```python
from build123d import *
from build123d.topology import SkipClean

# Parameters (mm, degrees)
BOSS_EXTRUDE1_DEPTH      = 1.3
BOSS_EXTRUDE2_DEPTH      = 10
BOSS_EXTRUDE2_DEPTH_BACK = 2.3
SKETCH2_R                = 1.79
SKETCH4_W                = 8.8
SKETCH4_H                = 1.3
BOSS_EXTRUDE4_DEPTH      = 2.4
SKETCH3_W                = 8.8
SKETCH3_H                = 10
BOSS_EXTRUDE3_DEPTH      = 1.3
FILLET4_R                = 1.3
FILLET6_R                = 1
SKETCH5_R                = 1.5
CUT_EXTRUDE1_DEPTH       = 2.4
FILLET7_R                = 1
FILLET4_OF_MIRROR1_R     = 1.3
FILLET6_OF_MIRROR1_R     = 1
FILLET7_OF_MIRROR1_R     = 1
BOSS_EXTRUDE5_START      = 7
SKETCH6_W                = 18
SKETCH6_H                = 70
SKETCH6_R                = 1.5
BOSS_EXTRUDE5_DEPTH      = 7
SKETCH9_R                = 4
CUT_EXTRUDE3_DEPTH       = 3
CUT_EXTRUDE4_DEPTH       = 72.965296541


with BuildPart() as part:
    # Sketch1 → Boss-Extrude1 (new body)
    with BuildSketch(Plane.XY):
        with BuildLine():
            Line((-4.7625, -4.5), (4.7625, -4.5))
            ThreePointArc((4.7625, -4.5), (8.887505516, 1.798424168), (1.465384615, 3.062520227))
            ThreePointArc((1.465384615, 3.062520227), (0, 2.423640328), (-1.465384615, 3.062520227))
            ThreePointArc((-1.465384615, 3.062520227), (-8.887505516, 1.798424168), (-4.7625, -4.5))
        make_face()
    boss_extrude1 = extrude(amount=BOSS_EXTRUDE1_DEPTH)

    # Sketch2 → Boss-Extrude2 (add, two sides: drawn at the far end of the back side and taken through both)
    with BuildSketch(Plane.XY.offset(1.3).offset(-BOSS_EXTRUDE2_DEPTH_BACK)):
        with Locations((-4.7625, 0)):
            Circle(SKETCH2_R)
        with Locations((4.7625, 0)):
            Circle(SKETCH2_R)
    extrude(amount=BOSS_EXTRUDE2_DEPTH + BOSS_EXTRUDE2_DEPTH_BACK)

    # Sketch4 → Boss-Extrude4 (add)
    with BuildSketch(Plane.XZ.offset(4.5)):
        with Locations((0, 0.65)):
            Rectangle(SKETCH4_W, SKETCH4_H)
    boss_extrude4 = extrude(amount=BOSS_EXTRUDE4_DEPTH)

    # Sketch3 → Boss-Extrude3 (add)
    with BuildSketch(Plane.XZ.offset(6.9)):
        with Locations((0, -3.7)):
            Rectangle(SKETCH3_W, SKETCH3_H)
    boss_extrude3 = extrude(amount=-BOSS_EXTRUDE3_DEPTH)

    # Fillet4
    fillet4_edges = [part.edges().sort_by_distance(p)[0] for p in [
        (0, -6.9, 1.3),
    ]]
    fillet(fillet4_edges, radius=FILLET4_R)

    # Fillet6
    fillet6_edges = [part.edges().sort_by_distance(p)[0] for p in [
        (0, -5.6, 0),
    ]]
    fillet(fillet6_edges, radius=FILLET6_R)

    # Sketch5 → Cut-Extrude1 (cut)
    with BuildSketch(Plane.XZ.offset(6.9)):
        with Locations(Location((0, -4.35, 0), (0, 0, 270))):
            Circle(SKETCH5_R)
    cut_extrude1 = extrude(amount=-CUT_EXTRUDE1_DEPTH, mode=Mode.SUBTRACT)

    # Fillet7
    fillet7_edges = [part.edges().sort_by_distance(p)[0] for p in [
        (-4.4, -6.25, -8.7),
        (4.4, -6.25, -8.7),
    ]]
    fillet(fillet7_edges, radius=FILLET7_R)

    # Mirror1: Boss-Extrude1, Boss-Extrude4, Boss-Extrude3, Cut-Extrude1 across plane
    add(boss_extrude1.mirror(Plane(origin=(0, 0, 5.15), x_dir=(1, 0, 0), z_dir=(0, 0, -1))))
    add(boss_extrude4.mirror(Plane(origin=(0, 0, 5.15), x_dir=(1, 0, 0), z_dir=(0, 0, -1))))
    add(boss_extrude3.mirror(Plane(origin=(0, 0, 5.15), x_dir=(1, 0, 0), z_dir=(0, 0, -1))))
    add(cut_extrude1.mirror(Plane(origin=(0, 0, 5.15), x_dir=(1, 0, 0), z_dir=(0, 0, -1))), mode=Mode.SUBTRACT)

    # Fillet4 of Mirror1
    fillet4_of_mirror1_edges = [part.edges().sort_by_distance(p)[0] for p in [
        (0, -6.9, 9),
    ]]
    fillet(fillet4_of_mirror1_edges, radius=FILLET4_OF_MIRROR1_R)

    # Fillet6 of Mirror1
    fillet6_of_mirror1_edges = [part.edges().sort_by_distance(p)[0] for p in [
        (0, -5.6, 10.3),
    ]]
    fillet(fillet6_of_mirror1_edges, radius=FILLET6_OF_MIRROR1_R)

    # Fillet7 of Mirror1
    fillet7_of_mirror1_edges = [part.edges().sort_by_distance(p)[0] for p in [
        (-4.4, -6.25, 19),
        (4.4, -6.25, 19),
    ]]
    fillet(fillet7_of_mirror1_edges, radius=FILLET7_OF_MIRROR1_R)

    # Sketch6 → Boss-Extrude5 (add)
    with SkipClean():  # the faces are left unmerged after this step: merging them gives an invalid solid
        with BuildSketch(Plane.XZ.offset(6.9).offset(BOSS_EXTRUDE5_START)):
            with Locations((0, 5.15)):
                Rectangle(SKETCH6_W, SKETCH6_H)
            with Locations(Location((0, 14.65, 0), (0, 0, 270))):
                Circle(SKETCH6_R, mode=Mode.SUBTRACT)
            with Locations(Location((0, -4.35, 0), (0, 0, 270))):
                Circle(SKETCH6_R, mode=Mode.SUBTRACT)
        extrude(amount=-BOSS_EXTRUDE5_DEPTH)

    # Sketch9 → Cut-Extrude3 (cut)
    with SkipClean():  # the faces are left unmerged after this step: merging them gives an invalid solid
        with BuildSketch(Plane.XZ.offset(13.9)):
            with Locations(Location((0, 14.65, 0), (0, 0, 270))):
                Circle(SKETCH9_R)
            with Locations(Location((0, -4.35, 0), (0, 0, 270))):
                Circle(SKETCH9_R)
        extrude(amount=-CUT_EXTRUDE3_DEPTH, mode=Mode.SUBTRACT)

    # Sketch11 → Cut-Extrude4 (cut, through all)
    with SkipClean():  # the faces are left unmerged after this step: merging them gives an invalid solid
        with BuildSketch(Plane.XY.offset(40.15)):
            Polygon((9, -12.432975638), (7.875, -13.9), (6.75, -12.432975638), (5.625, -13.9), (4.5, -12.432975638), (3.375, -13.9), (2.25, -12.432975638), (1.125, -13.9), (0, -12.432975638), (-1.125, -13.9), (-2.25, -12.432975638), (-3.375, -13.9), (-4.5, -12.432975638), (-5.625, -13.9), (-6.75, -12.432975638), (-7.875, -13.9), (-9, -12.432975638), (-9, -14.9), (9, -14.9), align=None)
        extrude(amount=-CUT_EXTRUDE4_DEPTH, mode=Mode.SUBTRACT)


solid = part.part
```
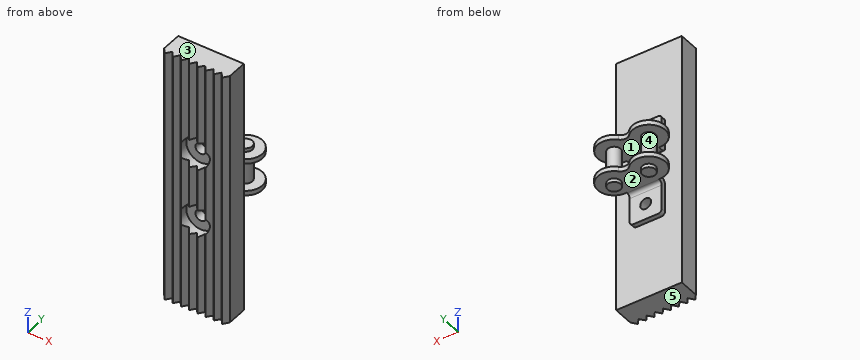
Build history of the part. All positions in model axes, mm. Face numbers are marked on the shaded views. A direction names the side the tool comes from. Coordinates: 2 decimals unless noted, no trailing zeros. Write each loop counter-clockwise with the first axis right and the second up, starting at its lowest first coordinate (ties: lowest second). Pieces come first, ordered by that corner, then holes.
1. Band-saw the part on B-B, the plane z = 26.5. Give the cut face in (x, y) (3 decimals).
Answer block:
outline: (-9, -12.433) - (-7.875, -13.9) - (-6.75, -12.433) - (-5.625, -13.9) - (-4.5, -12.433) - (-3.375, -13.9) - (-2.25, -12.433) - (-1.125, -13.9) - (0, -12.433) - (1.125, -13.9) - (2.25, -12.433) - (3.375, -13.9) - (4.5, -12.433) - (5.625, -13.9) - (6.75, -12.433) - (7.875, -13.9) - (9, -12.433) - (9, -6.9) - (-9, -6.9) - close
2. Band-saw the part on D-D, the plane z = 15. Give the cut face in (x, y) (3 decimals).
Answer block:
outline: (-9, -12.433) - (-7.875, -13.9) - (-6.75, -12.433) - (-5.625, -13.9) - (-4.5, -12.433) - (-3.985, -13.105) - (-3.985, -10.9) - (-1.459, -10.9) - (-1.459, -5.6) - (-4.4, -5.6) - (-4.4, -6.9) - (-9, -6.9) - close; (1.459, -10.9) - (3.985, -10.9) - (3.985, -13.105) - (4.5, -12.433) - (5.625, -13.9) - (6.75, -12.433) - (7.875, -13.9) - (9, -12.433) - (9, -6.9) - (4.4, -6.9) - (4.4, -5.6) - (1.459, -5.6) - close
3. Pull direction X, two halves, no side cores. Call the marked faces 4 and 5: released by +X, released by -X, zero draft, split by the parting line, or undercut.
Answer block:
face 4: undercut
face 5: zero draft
4. Drop flat-ended pins along their axis: pin 1 (1.8 mm diameter, centred on x = 0, z = 14.65, fed in from -Y); pin 2 (1.1 mm diameter, centred on x = -4.5, y = 0, fed in from +Z); pin 3 (0.6 mm diameter, centred on x = -1, y = -6, fed in from +Z); pin 4 (1.7 mm diameter, centred on y = -9.5, z = -3.5, fed in from +X). Give the stop position or say it passes through.
Answer block:
pin 1: passes through
pin 2: stops at z = 11.3
pin 3: stops at z = 19
pin 4: stops at x = 9
5. Drill centre lines: probe 1 along Z at (x, y) = (0, -11.6); probe 2 along Z at (x, y) = (-6.75, -2.5); probe 3 along X at (y, z) = (-11.75, -4.35). Where is each one in solid material? Low to high.
Answer block:
probe 1: z = -29.85 to -8.35, -0.35 to 10.65, 18.65 to 40.15
probe 2: z = 0 to 1.3, 9 to 10.3
probe 3: x = -9 to -4, 4 to 9
6. Band-saw the part on C-C, the plane z = -4.35. Give the cut face in (x, y) (3 decimals).
Answer block:
outline: (-9, -12.433) - (-7.875, -13.9) - (-6.75, -12.433) - (-5.625, -13.9) - (-4.5, -12.433) - (-4, -13.085) - (-4, -10.9) - (-1.5, -10.9) - (-1.5, -5.6) - (-4.4, -5.6) - (-4.4, -6.9) - (-9, -6.9) - close; (1.5, -10.9) - (4, -10.9) - (4, -13.085) - (4.5, -12.433) - (5.625, -13.9) - (6.75, -12.433) - (7.875, -13.9) - (9, -12.433) - (9, -6.9) - (4.4, -6.9) - (4.4, -5.6) - (1.5, -5.6) - close
7. 3-axis set-ups, long thin cutter, end or side, ignore diameter. For the marked faces 1, 2 and 3: which of +Z, -Z, +X, -X, +Y, -Y reach the whole face in a straight line?
Answer block:
face 1: none
face 2: -Z
face 3: +Z, +X, -X, +Y, -Y
